Check sheet for the drawn part. Datum: minimum x, y, z corner. Units: mm. A direction names the side the tool comes from. Coordinates: 2 decimals unless noted, no trailing zeros. Write each loop counter-clockwise with the first axis right and the second up, starting at its lowest first coordinate (ties: lowest second). Pieces come first, ordered by that corner, then holes. Notation, with made-up numbers: (-37.5, -16.5) -> (3.5, -16.5) arc R23 ccw to (3.5, -5.5) -> close; hole circle Ø8 at (41.25, 19.25). An arc over 180 degrees is marked (long way). Answer in a Markdown table with one row per item. Add a question column.
1. Cross-section at B-B on x = 9.5. Record the cut outline in (y, z) (3 decimals).
2. Mould release check, pull along Z, two halves, no side actions. Record for the marked faces 1, 2 and 3: pulls with the +Z half, pulls with the -Z half, needs draft (parallel to the pull), parting line crosses it, or undercut.
3. Set-up check for the marked faces 4, 5 and 6: record each of +Z, -Z, +X, -X, +Y, -Y from which the full face is reachable in a straight line by a thin tool's end or side.
4. Scan lines: L1, parallel to X at y = 1.6, z = 6.35 (3 decimals); L2, parallel to X at y = 0.9, z = 19.05 (3 decimals); L3, parallel to X at y = 2.95, z = 22.5 (3 decimals). Record each from-to range of solid material in increasing order. Write a range as from..to.
5. Depth check by flat-ended pin: P1, Ø1, axis at y = 1.5, z = 20, coming from the +X side (3 decimals); P2, Ø1.6, axis at x = 2.5, y = 2, coming from the +Z side. Enter the tip coordinate at first touch or a pass-through.
6. Cross-section at A-A on z = 6.35. Record the cut outline in (x, y) (3 decimals), and give its area (3 significant figures).
7. Cross-section at C-C on z = 19.05. Record the cut outline in (x, y) (3 decimals), and give its area (3 significant figures).
8. Cross-section at D-D on y = 1. Record the cut outline in (x, z) (3 decimals).
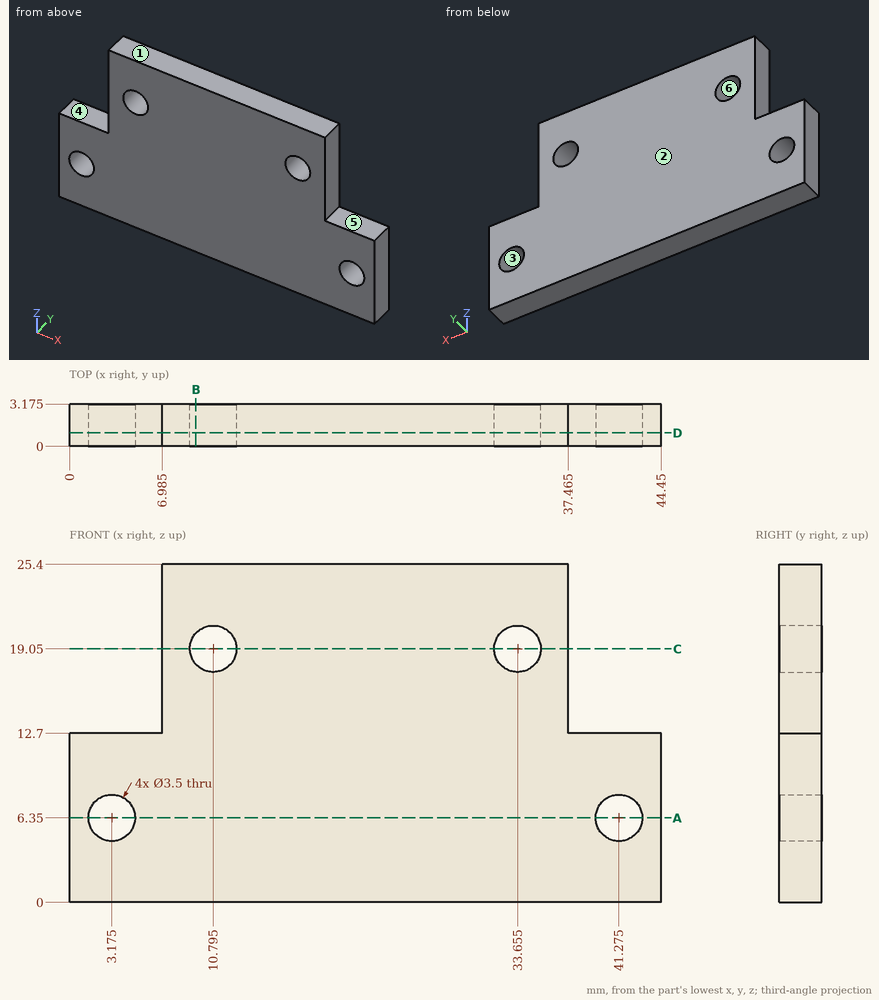
Results found:
| question | item | result |
|---|---|---|
| 1 | outline | (0, 0) -> (3.175, 0) -> (3.175, 17.873) -> (0, 17.873) -> close; (0, 20.227) -> (3.175, 20.227) -> (3.175, 25.4) -> (0, 25.4) -> close |
| 2 | face 1 | pulls with the +Z half |
| 2 | face 2 | needs draft |
| 2 | face 3 | undercut |
| 3 | face 4 | +Z, -X, +Y, -Y |
| 3 | face 5 | +Z, +X, +Y, -Y |
| 3 | face 6 | +Y, -Y |
| 4 | L1 | x = 0..1.425, 4.925..39.525, 43.025..44.45 |
| 4 | L2 | x = 6.985..9.045, 12.545..31.905, 35.405..37.465 |
| 4 | L3 | x = 6.985..37.465 |
| 5 | P1 | stops at x = 37.465 |
| 5 | P2 | stops at z = 12.7 |
| 6 | outline | (0, 0) -> (1.425, 0) -> (1.425, 3.175) -> (0, 3.175) -> close; (4.925, 0) -> (39.525, 0) -> (39.525, 3.175) -> (4.925, 3.175) -> close; (43.025, 0) -> (44.45, 0) -> (44.45, 3.175) -> (43.025, 3.175) -> close |
| 6 | area | 119 mm^2 |
| 7 | outline | (6.985, 0) -> (9.045, 0) -> (9.045, 3.175) -> (6.985, 3.175) -> close; (12.545, 0) -> (31.905, 0) -> (31.905, 3.175) -> (12.545, 3.175) -> close; (35.405, 0) -> (37.465, 0) -> (37.465, 3.175) -> (35.405, 3.175) -> close |
| 7 | area | 74.5 mm^2 |
| 8 | outline | (0, 0) -> (44.45, 0) -> (44.45, 12.7) -> (37.465, 12.7) -> (37.465, 25.4) -> (6.985, 25.4) -> (6.985, 12.7) -> (0, 12.7) -> close; hole circle Ø3.5 at (3.175, 6.35); hole circle Ø3.5 at (10.795, 19.05); hole circle Ø3.5 at (33.655, 19.05); hole circle Ø3.5 at (41.275, 6.35) |
